Print and shaded views of the part. All mm, measured from the part's lowest x, y and z. A direction names the side the tool comes from. Round coordinates to 2 decimals unless told otherwise and drop trailing zeros. Loops run counter-clockwise (first coordinate to the right, second up) from the corner with the lowest first, then second, coordinate; pieces in that order, holes last. Notation, with made-up numbers: (-19.75, -20.75) - (32.25, -20.75) arc R19 ccw to (32.25, 6.25) - close; hole circle Ø9 at (89, -6.5). An arc over 180 degrees is marked (long way). Use one line per item in the form item = value. Start each with the question number.
Q1. Mould opens along X. For the marked faces 3, 4 and 5 say: released by +X, released by -X, zero draft, split by the parting line, or undercut.
Q2. Saw through at C-C (y = 4). Count the separate pieces of the cut face and the enclosed holes in it, then the cut area to 3 significant figures.
Q3. Pin check, flat tips, straight feed: pin 1 (9 mm diameter, centred on y = 11.5, z = 23.5, fed in from +X); pin 2 (10 mm diameter, centred on x = 31, y = 5, fed in from +Z). Stop position of each tip, or through.
Q4. Drill centre lines: line 1 (Z direction, x = 8.89, y = 8); line 2 (X direction, y = 14.25, z = 35.56); line 3 (X direction, y = 7.25, z = 13). Where is each one in solid material? Low to high.
Q5. 3-axis set-ups, long thin cutter, end or side, ignore diameter. For the marked faces 1 and 2: which of +Z, -Z, +X, -X, +Y, -Y reach the whole face in a straight line?
Q6. Saw through at D-D (z = 19). Give the cut face in (x, y).
Q7. Saw through at A-A (x = 8.89). Give the cut face in (y, z), then the cut area to 3 significant figures.
Q8. Saw through at B-B (z = 35.56). Give the cut face in (x, y).
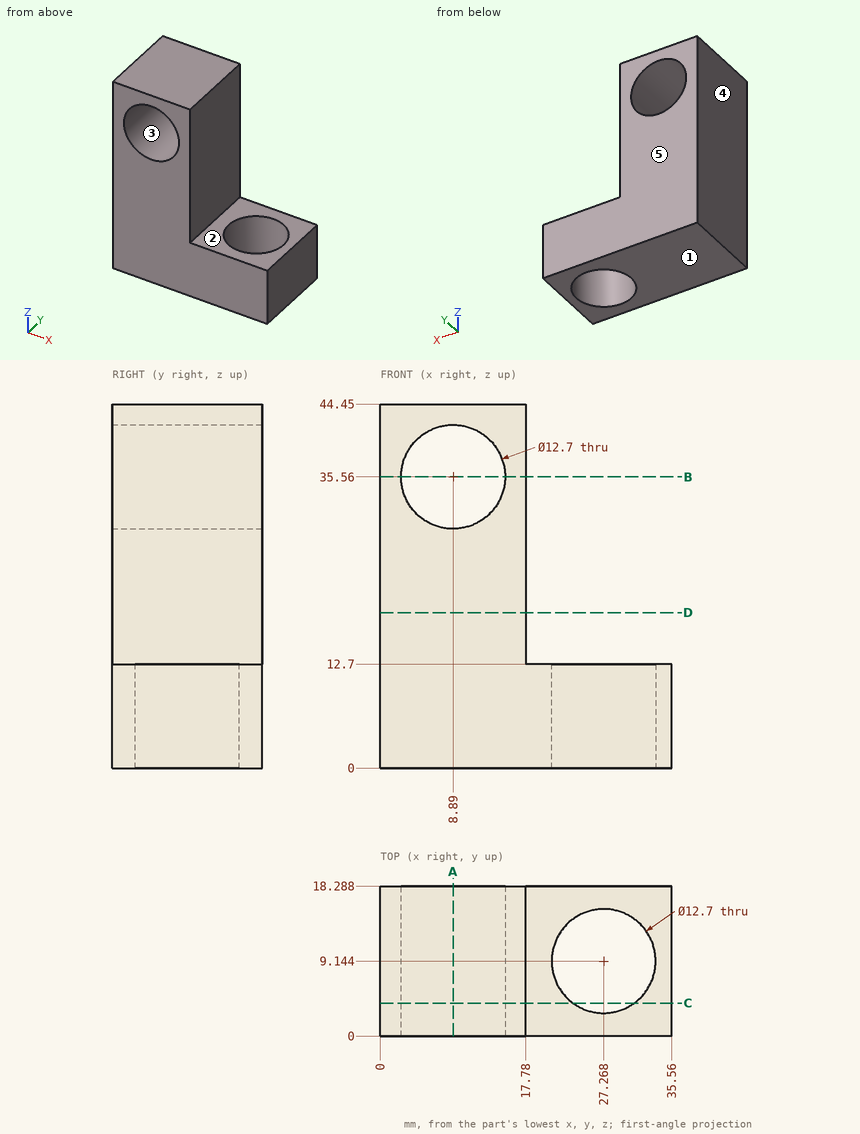
Report:
q1.face_3 = undercut
q1.face_4 = released by -X
q1.face_5 = zero draft
q2.separate_pieces = 2
q2.enclosed_holes = 1
q2.area = 795 mm²
q3.pin_1 = 17.78
q3.pin_2 = 12.7
q4.line_1 = 0 to 29.21, 41.91 to 44.45
q4.line_2 = 0 to 2.54, 15.24 to 17.78
q4.line_3 = 0 to 17.78
q5.face_1 = -Z, +X, -X, +Y, -Y
q5.face_2 = +Z, +X, +Y, -Y
q6.outline = (0, 0) - (17.78, 0) - (17.78, 18.29) - (0, 18.29) - close
q7.outline = (0, 0) - (18.29, 0) - (18.29, 29.21) - (0, 29.21) - close; (0, 41.91) - (18.29, 41.91) - (18.29, 44.45) - (0, 44.45) - close
q7.area = 581 mm²
q8.outline = (0, 0) - (2.54, 0) - (2.54, 18.29) - (0, 18.29) - close; (15.24, 0) - (17.78, 0) - (17.78, 18.29) - (15.24, 18.29) - close
